For this review, take the finished solid that the model builds, in its own axes (mm). A direction names the side the tool comes from. Give positions to 0.01 mm unless a question says otherwise; leave off trailing zeros. Write each loop counter-clockwise with the first axis right and the second up, starting at its lowest first coordinate (ties: lowest second). Pieces come first, ordered by that corner, then holes. Notation, with made-up numbers: (-16, 49) -> (36, 49) arc R7 ccw to (36, 60) -> close; hole circle Ø9 at (-9, 84). An arc over 180 degrees is marked (long way). Return JSON: item names as keys, results as strings.
from build123d import *

# Parameters (mm, degrees)
ESQUISSE1_R        = 10
ESQUISSE1_R_2      = 3.5
BOSS_EXTRU_1_DEPTH = 4
BOSS_EXTRU_2_START = 10
ESQUISSE2_R        = 10
ESQUISSE2_R_2      = 6.75
BOSS_EXTRU_2_DEPTH = 10
BOSS_EXTRU_3_START = 1.5
BOSS_EXTRU_3_DEPTH = 1.5
CONG_1_R           = 2
BOSS_EXTRU_6_START = -2
ESQUISSE13_R       = 3.5
BOSS_EXTRU_6_DEPTH = 2
ESQUISSE15_R       = 10
BOSS_EXTRU_7_DEPTH = 2
ESQUISSE21_R       = 3
BOSS_EXTRU_8_DEPTH = 30


with BuildPart() as part:
    # Esquisse1 → Boss.-Extru.1 (new body)
    with BuildSketch(Plane(origin=(0, 0, 0), x_dir=(1, 0, 0), z_dir=(0, 1, 0))):
        with Locations(Location((0, 0, 0), (0, 0, 270))):
            Circle(ESQUISSE1_R)
        with Locations(Location((0, 0, 0), (0, 0, 270))):
            Circle(ESQUISSE1_R_2, mode=Mode.SUBTRACT)
    extrude(amount=BOSS_EXTRU_1_DEPTH)

    # Esquisse2 → Boss.-Extru.2 (add)
    with BuildSketch(Plane.XZ.offset(BOSS_EXTRU_2_START)):
        with Locations(Location((0, 0, 0), (0, 0, 270))):
            Circle(ESQUISSE2_R)
        with Locations(Location((0, 0, 0), (0, 0, 270))):
            Circle(ESQUISSE2_R_2, mode=Mode.SUBTRACT)
    extrude(amount=-BOSS_EXTRU_2_DEPTH)

    # Esquisse5 → Révolution2 (revolve)
    with BuildSketch(Plane(origin=(0, 0, 0), x_dir=(0, 0, -1), z_dir=(1, 0, 0))):
        Polygon((-10, -10), (-6.75, -10), (-6.250000000000001, -10.499999999999995), (-9.500000000000004, -10.499999999999993), align=None)
    revolve(axis=Axis((0, 0, 0), (0, -1, 0)))

    # Esquisse7 → Boss.-Extru.3 (add)
    with BuildSketch(Plane.XZ.offset(BOSS_EXTRU_3_START)):
        with BuildLine():
            ThreePointArc((-3.471641565041511, 0.4446401285040917), (-3.3915764747476542, 0.8644125264815606), (-3.260950790974577, 1.2712985246755686))
            Line((-3.260950790974577, 1.2712985246755686), (-6.288976525451004, 2.4517900118742246))
            ThreePointArc((-6.288976525451004, 2.4517900118742246), (-6.54089748701339, 1.6670813010714052), (-6.695308732580065, 0.8575202478290395))
            Line((-6.695308732580065, 0.8575202478290395), (-3.471641565041511, 0.4446401285040917))
        make_face()
        with BuildLine():
            ThreePointArc((-0.44464012850385526, -3.47164156504154), (-0.8644125264814398, -3.3915764747476906), (-1.2712985246755584, -3.2609507909745816))
            Line((-1.271298524675558, -3.2609507909745803), (-2.4517900118740936, -6.288976525450949))
            ThreePointArc((-2.4517900118740936, -6.28897652545095), (-1.6670813010712728, -6.54089748701333), (-0.8575202478289087, -6.69530873258001))
            Line((-0.8575202478289086, -6.695308732580009), (-0.4446401285038535, -3.4716415650415393))
        make_face()
        with BuildLine():
            ThreePointArc((3.4716415650415344, -0.44464012850390167), (3.391576474747708, -0.8644125264813738), (3.2609507909746505, -1.271298524675382))
            Line((3.2609507909746522, -1.2712985246753834), (6.288976525451078, -2.4517900118740386))
            ThreePointArc((6.288976525451079, -2.451790011874039), (6.540897487013439, -1.6670813010712129), (6.69530873258014, -0.8575202478288542))
            Line((6.6953087325801395, -0.8575202478288538), (3.471641565041585, -0.4446401285039065))
        make_face()
        with BuildLine():
            Line((0.857520247828984, 6.6953087325801945), (0.44464012850403645, 3.4716415650416406))
            ThreePointArc((0.44464012850402057, 3.4716415650415193), (0.8644125264815102, 3.391576474747673), (1.2712985246755357, 3.2609507909745905))
            Line((1.2712985246755355, 3.26095079097459), (2.4517900118741687, 6.288976525451134))
            ThreePointArc((2.4517900118741687, 6.288976525451133), (1.6670813010713434, 6.540897487013499), (0.857520247828984, 6.6953087325801945))
        make_face()
    extrude(amount=-BOSS_EXTRU_3_DEPTH)

    # Congé1
    # the kernel refuses this fillet: 2 mm, written as the material it adds along each edge
    with BuildSketch(Plane(origin=(-11.497312291654126, 0, 1.472550180954296), x_dir=(-0.1270400367153696, 0, -0.9918975900118709), z_dir=(0.9918975900118709, 0, -0.1270400367153696))) as cong_1_piece_1_section:
        with BuildLine():
            CenterArc((1.9364916731037083, -2), CONG_1_R, 90, 75.5224878140701)
            Line((-2.2e-16, -1.5), (0, 0))
            Line((0, 0), (1.9364916731037083, 0))
        make_face()
    cong_1_piece_1 = extrude(amount=12.932458365518517, mode=Mode.PRIVATE)
    cong_1_piece_1 = cong_1_piece_1 - Plane(origin=(0, 0, 0), x_dir=(-1.8e-16, 0, 1), z_dir=(0, -1, 0)) * Cylinder(3.5, 34, mode=Mode.PRIVATE)
    cong_1_piece_1 = cong_1_piece_1 & Plane(origin=(0, 0, 0), x_dir=(-1.8e-16, 0, -1), z_dir=(0, -1, 0)) * Cylinder(6.75, 34, mode=Mode.PRIVATE)
    add(cong_1_piece_1)
    with BuildSketch(Plane(origin=(1.2496235326849163, 0, -0.4871721946552088), x_dir=(0.3632281499072788, 0, 0.9317002259927467), z_dir=(-0.9317002259927468, 0, 0.3632281499072788))) as cong_1_piece_2_section:
        with BuildLine():
            CenterArc((1.9364916731037085, -2), CONG_1_R, 90, 75.5224878140701)
            Line((0, -1.5), (0, 0))
            Line((0, 0), (1.9364916731037085, 0))
        make_face()
    cong_1_piece_2 = extrude(amount=12.932458365518542, mode=Mode.PRIVATE)
    cong_1_piece_2 = cong_1_piece_2 - Plane(origin=(0, 0, 0), x_dir=(-1.8e-16, 0, 1), z_dir=(0, -1, 0)) * Cylinder(3.5, 34, mode=Mode.PRIVATE)
    cong_1_piece_2 = cong_1_piece_2 & Plane(origin=(0, 0, 0), x_dir=(-1.8e-16, 0, -1), z_dir=(0, -1, 0)) * Cylinder(6.75, 34, mode=Mode.PRIVATE)
    add(cong_1_piece_2)
    with BuildSketch(Plane(origin=(-1.4725501809543382, 0, -11.497312291654048), x_dir=(0.9918975900118664, 0, -0.12704003671540534), z_dir=(0.12704003671540534, 0, 0.9918975900118664))) as cong_1_piece_3_section:
        with BuildLine():
            CenterArc((1.9364916731037087, -2.0000000000000004), CONG_1_R, 90, 75.5224878140701)
            Line((0, -1.5000000000000004), (0, 0))
            Line((0, 0), (1.9364916731037087, 0))
        make_face()
    cong_1_piece_3 = extrude(amount=12.932458365518444, mode=Mode.PRIVATE)
    cong_1_piece_3 = cong_1_piece_3 - Plane(origin=(0, 0, 0), x_dir=(-1.8e-16, 0, 1), z_dir=(0, -1, 0)) * Cylinder(3.5, 34, mode=Mode.PRIVATE)
    cong_1_piece_3 = cong_1_piece_3 & Plane(origin=(0, 0, 0), x_dir=(-1.8e-16, 0, -1), z_dir=(0, -1, 0)) * Cylinder(6.75, 34, mode=Mode.PRIVATE)
    add(cong_1_piece_3)
    with BuildSketch(Plane(origin=(0.4871721946550931, 0, 1.2496235326849625), x_dir=(-0.9317002259927569, 0, 0.3632281499072527), z_dir=(-0.3632281499072527, 0, -0.931700225992757))) as cong_1_piece_4_section:
        with BuildLine():
            CenterArc((1.9364916731037085, -2), CONG_1_R, 90, 75.5224878140701)
            Line((0, -1.5), (0, 0))
            Line((0, 0), (1.9364916731037085, 0))
        make_face()
    cong_1_piece_4 = extrude(amount=12.932458365518446, mode=Mode.PRIVATE)
    cong_1_piece_4 = cong_1_piece_4 - Plane(origin=(0, 0, 0), x_dir=(-1.8e-16, 0, 1), z_dir=(0, -1, 0)) * Cylinder(3.5, 34, mode=Mode.PRIVATE)
    cong_1_piece_4 = cong_1_piece_4 & Plane(origin=(0, 0, 0), x_dir=(-1.8e-16, 0, -1), z_dir=(0, -1, 0)) * Cylinder(6.75, 34, mode=Mode.PRIVATE)
    add(cong_1_piece_4)
    with BuildSketch(Plane(origin=(11.4973122916542, 0, -1.4725501809541097), x_dir=(0.12704003671536943, 0, 0.9918975900118709), z_dir=(-0.991897590011871, 0, 0.12704003671536945))) as cong_1_piece_5_section:
        with BuildLine():
            CenterArc((1.9364916731037083, -2.0000000000000004), CONG_1_R, 90, 75.5224878140701)
            Line((-2.2e-16, -1.5000000000000004), (0, 0))
            Line((0, 0), (1.9364916731037083, 0))
        make_face()
    cong_1_piece_5 = extrude(amount=12.932458365518519, mode=Mode.PRIVATE)
    cong_1_piece_5 = cong_1_piece_5 - Plane(origin=(0, 0, 0), x_dir=(-1.8e-16, 0, 1), z_dir=(0, -1, 0)) * Cylinder(3.5, 34, mode=Mode.PRIVATE)
    cong_1_piece_5 = cong_1_piece_5 & Plane(origin=(0, 0, 0), x_dir=(-1.8e-16, 0, -1), z_dir=(0, -1, 0)) * Cylinder(6.75, 34, mode=Mode.PRIVATE)
    add(cong_1_piece_5)
    with BuildSketch(Plane(origin=(-1.2496235326848435, 0, 0.4871721946553944), x_dir=(-0.3632281499072787, 0, -0.9317002259927468), z_dir=(0.9317002259927469, 0, -0.3632281499072787))) as cong_1_piece_6_section:
        with BuildLine():
            CenterArc((1.936491673103709, -2), CONG_1_R, 90, 75.5224878140701)
            Line((2.1e-16, -1.5), (0, 0))
            Line((0, 0), (1.936491673103709, 0))
        make_face()
    cong_1_piece_6 = extrude(amount=12.932458365518547, mode=Mode.PRIVATE)
    cong_1_piece_6 = cong_1_piece_6 - Plane(origin=(0, 0, 0), x_dir=(-1.8e-16, 0, 1), z_dir=(0, -1, 0)) * Cylinder(3.5, 34, mode=Mode.PRIVATE)
    cong_1_piece_6 = cong_1_piece_6 & Plane(origin=(0, 0, 0), x_dir=(-1.8e-16, 0, -1), z_dir=(0, -1, 0)) * Cylinder(6.75, 34, mode=Mode.PRIVATE)
    add(cong_1_piece_6)
    with BuildSketch(Plane(origin=(1.4725501809542403, 0, 11.497312291654257), x_dir=(-0.9918975900118709, 0, 0.1270400367153695), z_dir=(-0.1270400367153695, 0, -0.9918975900118709))) as cong_1_piece_7_section:
        with BuildLine():
            CenterArc((1.936491673103709, -2), CONG_1_R, 90, 75.5224878140701)
            Line((2.2e-16, -1.5), (0, 0))
            Line((0, 0), (1.936491673103709, 0))
        make_face()
    cong_1_piece_7 = extrude(amount=12.93245836551852, mode=Mode.PRIVATE)
    cong_1_piece_7 = cong_1_piece_7 - Plane(origin=(0, 0, 0), x_dir=(-1.8e-16, 0, 1), z_dir=(0, -1, 0)) * Cylinder(3.5, 34, mode=Mode.PRIVATE)
    cong_1_piece_7 = cong_1_piece_7 & Plane(origin=(0, 0, 0), x_dir=(-1.8e-16, 0, -1), z_dir=(0, -1, 0)) * Cylinder(6.75, 34, mode=Mode.PRIVATE)
    add(cong_1_piece_7)
    with BuildSketch(Plane(origin=(-0.4871721946551535, 0, -1.2496235326849385), x_dir=(0.9317002259927538, 0, -0.3632281499072605), z_dir=(0.36322814990726054, 0, 0.931700225992754))) as cong_1_piece_8_section:
        with BuildLine():
            CenterArc((1.9364916731037085, -2), CONG_1_R, 90, 75.5224878140701)
            Line((0, -1.5), (0, 0))
            Line((0, 0), (1.9364916731037085, 0))
        make_face()
    cong_1_piece_8 = extrude(amount=12.932458365518647, mode=Mode.PRIVATE)
    cong_1_piece_8 = cong_1_piece_8 - Plane(origin=(0, 0, 0), x_dir=(-1.8e-16, 0, 1), z_dir=(0, -1, 0)) * Cylinder(3.5, 34, mode=Mode.PRIVATE)
    cong_1_piece_8 = cong_1_piece_8 & Plane(origin=(0, 0, 0), x_dir=(-1.8e-16, 0, -1), z_dir=(0, -1, 0)) * Cylinder(6.75, 34, mode=Mode.PRIVATE)
    add(cong_1_piece_8)

    # Esquisse13 → Boss.-Extru.6 (add)
    with BuildSketch(Plane(origin=(0, 4, 0), x_dir=(1, 0, 0), z_dir=(0, 1, 0)).offset(BOSS_EXTRU_6_START)):
        with Locations(Location((0, 0, 0), (0, 0, 97.298580632))):
            Circle(ESQUISSE13_R)
    extrude(amount=BOSS_EXTRU_6_DEPTH)

    # Esquisse15 → Boss.-Extru.7 (add)
    with BuildSketch(Plane(origin=(0, 4, 0), x_dir=(1, 0, 0), z_dir=(0, 1, 0))):
        with Locations(Location((0, 0, 0), (0, 0, 90))):
            Circle(ESQUISSE15_R)
    extrude(amount=BOSS_EXTRU_7_DEPTH)

    # Esquisse21 → Boss.-Extru.8 (add)
    with BuildSketch(Plane(origin=(0, 6, 0), x_dir=(1, 0, 0), z_dir=(0, 1, 0))):
        with Locations(Location((0, 0, 0), (0, 0, 270))):
            Circle(ESQUISSE21_R)
    extrude(amount=BOSS_EXTRU_8_DEPTH)


solid = part.part
1. The part is to be moulded in two halves that separate along X. For faces 3 (the flat face through (6.2, -10.5, -2)), 4 (the flat face through (1, -1.5, 5)), 5 (the cylindrical face through (0.9, 20.79, 2.86)), say which applies: +X half, -X half, draft (parallel to the pull), parting line (faces both ways), or undercut.
Results found:
{"face 3": "draft", "face 4": "undercut", "face 5": "parting line"}
2. To check wall thickness, follow probe 1 along X at (y, z) = (-2.75, 0); probe 2 along X at (y, z) = (1.15, 0). State the ranges of each line that lie inside material, in increasing order.
Results found:
{"probe 1": "x = -10 to -6.75, 6.75 to 10", "probe 2": "x = -10 to -3.5, 3.5 to 10"}
3. For pin 1 (3 mm diameter, centred on x = 2, z = 7.5, fed in from +Y); pin 2 (10 mm diameter, centred on x = -3, z = -1, fed in from +Y); pin 3 (4 mm diameter, centred on x = 6.5, y = 30, fed in from +Z); pin 4 (1.6 mm diameter, centred on x = -4.5, z = 1.5, fed in from -Y), all flat-tipped, find the tip position at first contact; note any pin that passes through.
Results found:
{"pin 1": "stops at y = 6", "pin 2": "stops at y = 36", "pin 3": "passes through", "pin 4": "stops at y = -1.5"}
4. Add section B-B, the plane y = 18.5. State the section outline as (x, z) points.
Results found:
{"outline": "circle Ø6 at (0, 0)"}
5. Add section A-A, the plane y = -4.5. State the section outline as (x, z) points, plus the area to 3 significant figures.
Results found:
{"outline": "circle Ø20 at (0, 0); hole circle Ø13.5 at (0, 0)", "area": "171 mm²"}
6. For faces 1 (the flat face through (0, 36, 0)), 2 (the cylindrical face through (-2.42, -0.41, -4.21)), list the 3-axis set-ups (+Z, -Z, +X, -X, +Y, -Y) from which the entire face can be reached by the end or side of a thin tool; tool diameter is ignored.
Results found:
{"face 1": "+Z, -Z, +X, -X, +Y", "face 2": "none"}
